from build123d import *

# Parameters (mm, degrees)
PAD_DEPTH       = 20
SKETCH001_R     = 16
POCKET_DEPTH    = 10.5
SKETCH002_R     = 3.5
POCKET001_DEPTH = 10
FILLET_R        = 2
FILLET001_R     = 2
FILLET002_R     = 1
FILLET003_R     = 1


with BuildPart() as part:
    # Sketch → Pad (new body)
    with BuildSketch(Plane.XY):
        with BuildLine():
            Line((-50, -3), (-50, 3))
            Line((-50, 3), (-30.4, 3))
            ThreePointArc((-30.4, 3), (-24.229838, 6.236305), (-23.384615, 13.15224))
            ThreePointArc((23.384615, 13.15224), (0, 46.993041), (-23.384615, 13.15224))
            ThreePointArc((23.384615, 13.15224), (24.229838, 6.236305), (30.4, 3))
            Line((30.4, 3), (50, 3))
            Line((50, 3), (50, -3))
            Line((50, -3), (-50, -3))
        make_face()
    extrude(amount=PAD_DEPTH)

    # Sketch001 (on Face10 of Pad) → Pocket (cut)
    with BuildSketch(Plane.XY.offset(20)):
        with Locations((0, 22)):
            Circle(SKETCH001_R)
    extrude(amount=-POCKET_DEPTH, mode=Mode.SUBTRACT)

    # Sketch002 (on Face10 of Pocket) → Pocket001 (cut)
    with BuildSketch(Plane(origin=(0, 3, 0), x_dir=(-1, 0, 0), z_dir=(0, 1, 0))):
        with Locations((-40, 10)):
            Circle(SKETCH002_R)
        with Locations((40, 10)):
            Circle(SKETCH002_R)
    extrude(amount=-POCKET001_DEPTH, mode=Mode.SUBTRACT)

    # Fillet
    fillet_edges = [part.edges().sort_by_distance(p)[0] for p in [
        (0, 46.993041, 20),
    ]]
    fillet(fillet_edges, radius=FILLET_R)

    # Fillet001
    fillet001_edges = [part.edges().sort_by_distance(p)[0] for p in [
        (0, 46.993041, 0),
    ]]
    fillet(fillet001_edges, radius=FILLET001_R)

    # Fillet002
    fillet002_edges = [part.edges().sort_by_distance(p)[0] for p in [
        (-50, 3, 10),
    ]]
    fillet(fillet002_edges, radius=FILLET002_R)

    # Fillet003
    fillet003_edges = [part.edges().sort_by_distance(p)[0] for p in [
        (50, 3, 10),
    ]]
    fillet(fillet003_edges, radius=FILLET003_R)


solid = part.part
Work out the finished part from the listing and answer in its coordinate system (mm). A direction names the side the tool comes from. Give positions to 0.01 mm unless a question says otherwise; leave off trailing zeros. Order: outer loops, then holes, each group sorted by start corner. A loop starts at its lowest first (then second) coordinate and runs counter-clockwise, first axis right, second up. Notation, with made-up numbers: M -15.75,3 L 9.25,3 A32 cw 9.25,38 Z; hole C 47,76 d1. An arc over 180 degrees is marked long. Return JSON: item names as keys, results as strings.
Q1. The mould has two halves that part along X. Classify faces 1 (the face through (-24.29, 6.15, 9.89)), 2 (the face through (0, 22, 9.5)), 3 (the face through (-39.83, 2.4, 0.57)), 4 (the face through (-37.2, 0, 7.9)): pulls with the +X half, pulls with the -X half, needs draft (parallel to the pull), parting line crosses it, or undercut.
Answer below:
{"face 1": "pulls with the -X half", "face 2": "undercut", "face 3": "needs draft", "face 4": "undercut"}
Q2. Find the intervals of material crossed by line 1 along Z through (x, y) = (-40, -1); line 2 along Y through (x, z) = (0, 12.25); line 3 along Z through (x, y) = (-7.5, 19), in increasing order. Write a range as [from, to].
Answer below:
{"line 1": "z = [0, 6.5], [13.5, 20]", "line 2": "y = [-3, 6], [38, 46.99]", "line 3": "z = [0, 9.5]"}
Q3. Find section B-B, the plane z = 14.75. Write down the section's boundary in (x, y), and give its area (3 significant figures).
Answer below:
{"outline": "M -50,-3 L 50,-3 L 50,2 A1 ccw 49,3 L 30.4,3 A7.5 cw 23.38,13.15 A25 ccw long -23.38,13.15 A7.5 cw -30.4,3 L -49,3 A1 ccw -50,2 Z; hole C 0,22 d32", "area": "1,700 mm^2"}
Q4. Each of these flat-tipped pins is pushed along its axis until it touches: pin 1 (1 mm diameter, centred on x = 21.5, z = 17, fed in from +Y); pin 2 (9 mm diameter, centred on x = 40, z = 10, fed in from +Y); pin 3 (10 mm diameter, centred on x = -13, z = 16, fed in from +Y). Where does it stop, or does it pass through?
Answer below:
{"pin 1": "stops at y = 35.56", "pin 2": "stops at y = 3", "pin 3": "stops at y = 45.68"}
Q5. Which of the six approach directions +Z, -Z, +X, -X, +Y, -Y give full straight-line access (tool end or side, diameter ignored) to faces 5 (the face through (39.57, 2.4, 19.43)), 6 (the face through (-39.83, 2.4, 19.43)), 7 (the face through (40, 3, 6)), 8 (the face through (39.57, 2.4, 0.57))?
Answer below:
{"face 5": "+Z, +X, +Y", "face 6": "+Z, -X, +Y", "face 7": "+Z, -Z, +X, +Y", "face 8": "-Z, +X, +Y"}
Q6. Find section A-A, the plane x = 40. Write down the section's boundary in (y, z), and give its area (3 significant figures).
Answer below:
{"outline": "M -3,0 L 1,0 A2 ccw 3,2 L 3,6.5 L -3,6.5 Z; M -3,13.5 L 3,13.5 L 3,18 A2 ccw 1,20 L -3,20 Z", "area": "76.3 mm^2"}
Q7. Find section C-C, the plane x = 0. Write down the section's boundary in (y, z), and give its area (3 significant figures).
Answer below:
{"outline": "M -3,0 L 44.99,0 A2 ccw 46.99,2 L 46.99,18 A2 ccw 44.99,20 L 38,20 L 38,9.5 L 6,9.5 L 6,20 L -3,20 Z", "area": "662 mm^2"}
